```python
from build123d import *

# Parameters (mm, degrees)
F1_DEPTH = 2


with BuildPart() as f1:
    # F0 (on Top) → F1 (new body)
    with BuildSketch(Plane.XY):
        with BuildLine():
            Line((19.433085, 43.702438), (-23.47875, 43.702438))
            Line((-23.47875, 43.702438), (-23.47875, 25.546357))
            ThreePointArc((-23.47875, 25.546357), (-18.069214, 16.011021), (-21.1889, 5.501345))
            Line((-21.1889, 5.501345), (-21.1889, 2.342773))
            ThreePointArc((-21.1889, 2.342773), (-17.97875, -6.577941), (-21.1889, -15.498655))
            Line((-21.1889, -15.498655), (-21.1889, -18.657227))
            ThreePointArc((-21.1889, -18.657227), (-18.069214, -29.166902), (-23.47875, -38.702238))
            Line((-23.47875, -38.702238), (19.433085, -38.702238))
            Line((19.433085, -38.702238), (19.433085, 22.291379))
            ThreePointArc((19.433085, 22.291379), (15.933085, 31.922059), (19.433085, 41.55274))
            Line((19.433085, 41.55274), (19.433085, 43.702438))
        make_face()
    extrude(amount=F1_DEPTH)


solid = f1.part
```
Design review of the part built by this model. Coordinates are the model's own, in mm. A direction names the side the tool comes from. Round coordinates to 2 decimals unless told otherwise and drop trailing zeros. Order: outer loops, then holes, each group sorted by start corner. A loop starts at its lowest first (then second) coordinate and runs counter-clockwise, first axis right, second up. Notation, with made-up numbers: (33.5, 0) - (49.5, 0) arc R20 cw to (49.5, 8) - close; hole circle Ø11 at (-33, 52.25). An arc over 180 degrees is marked (long way). Return JSON: item names as keys, results as strings.
Q1. The part is to be moulded in two halves that separate along Y. For faces 1 (the flat face through (-2, 43.702, 1)), 2 (the cylindrical face through (15.934, 31.776, 0.986)), 3 (the flat face through (-2, 3, 0)), say which applies: pulls with the +Y half, pulls with the -Y half, needs draft (parallel to the pull), parting line crosses it, or undercut.
Computed values:
{"face 1": "pulls with the +Y half", "face 2": "undercut", "face 3": "needs draft"}
Q2. Consider section B-B on z = 1.15. Write out the cut boundary in (x, y).
Computed values:
{"outline": "(-23.48, -38.7) - (19.43, -38.7) - (19.43, 22.29) arc R15 cw to (19.43, 41.55) - (19.43, 43.7) - (-23.48, 43.7) - (-23.48, 25.55) arc R14 cw to (-21.19, 5.5) - (-21.19, 2.34) arc R14 cw to (-21.19, -15.5) - (-21.19, -18.66) arc R14 cw to start"}
Q3. For pin 1 Ø1 at (y, z) = (4, 1) entering from -X; pin 2 Ø1 at (y, z) = (23, 1.5) entering from -X, all flat-tipped, find the tip position at first contact; note any pin that passes through.
Computed values:
{"pin 1": "stops at x = -21.19", "pin 2": "stops at x = -21.32"}
Q4. Consider section D-D on y = 29.5. Write out the cut boundary in (x, z), plus the area to 3 significant figures.
Computed values:
{"outline": "(-23.48, 0) - (16.13, 0) - (16.13, 2) - (-23.48, 2) - close", "area": "79.2 mm2"}
Q5. Machinability: for faces 4 (the flat face through (-2, -38.702, 1)), 5 (the flat face through (-21.189, 4, 1)), which of the approach directions +Z, -Z, +X, -X, +Y, -Y give a long, thin tool a straight path to every point of the face, cutting with its end or side? Answer none if there is none.
Computed values:
{"face 4": "+Z, -Z, +X, -X, -Y", "face 5": "+Z, -Z, -X"}
Q6. Consider section C-C on y = 8. Write out the cut boundary in (x, z).
Computed values:
{"outline": "(-19.54, 0) - (19.43, 0) - (19.43, 2) - (-19.54, 2) - close"}
Q7. Wall thickness on L1, parallel to Y at x = 17, z = 0.4; L2, parallel to X at y = -16.5, z = 1.5; L3, parallel to X at y = 1, z = 0.4: over which ranges is each line inside the solid? List them lowest first. Write a range as [from, to].
Computed values:
{"L1": "y = [-38.7, 26.37], [37.48, 43.7]", "L2": "x = [-21.19, 19.43]", "L3": "x = [-20.21, 19.43]"}
Q8. Consider section A-A on x = 17.5. Write out the cut boundary in (y, z).
Computed values:
{"outline": "(-38.7, 0) - (25.25, 0) - (25.25, 2) - (-38.7, 2) - close; (38.6, 0) - (43.7, 0) - (43.7, 2) - (38.6, 2) - close"}
